Source: CAD feature listing. Evaluate the final solid. Frame: model axes, mm. A direction names the side the tool comes from. Round coordinates to 2 decimals unless told otherwise and drop trailing zeros. Write each loop counter-clockwise with the first axis right and the second up, starting at its lowest first coordinate (ties: lowest second). Pieces come first, ordered by that corner, then holes. Notation, with made-up numbers: (-11.5, -14) -> (5.5, -14) arc R28 ccw to (5.5, 12) -> close; hole circle Ø6 at (-15, 69). An arc over 180 degrees is marked (long way). Put each result on its own line as item: value.
```python
from build123d import *

# Parameters (mm, degrees)
SKETCH2_R          = 1.5875
CUT_EXTRUDE1_DEPTH = 13.7


with BuildPart() as part:
    # Sketch1 → Revolve1 (revolve)
    with BuildSketch(Plane.XY):
        with BuildLine():
            Line((12.7, 25.4), (17.4625, 25.4))
            ThreePointArc((17.4625, 25.4), (18.585032015, 24.935032015), (19.05, 23.8125))
            Line((19.05, 23.8125), (19.05, 14.2875))
            ThreePointArc((19.05, 14.2875), (19.514967985, 13.164967985), (20.6375, 12.7))
            Line((20.6375, 12.7), (33.3375, 12.7))
            ThreePointArc((33.3375, 12.7), (34.460032015, 12.235032015), (34.925, 11.1125))
            Line((34.925, 11.1125), (34.925, 0))
            Line((34.925, 0), (25.4, 0))
            Line((25.4, 0), (25.4, 3.175))
            ThreePointArc((25.4, 3.175), (24.47006403, 5.42006403), (22.225, 6.35))
            Line((22.225, 6.35), (12.7, 6.35))
            Line((12.7, 6.35), (12.7, 25.4))
        make_face()
    revolve(axis=Axis((0, 0, 0), (0, 1, 0)))

    # Sketch2 → Cut-Extrude1 (cut, through all)
    with BuildSketch(Plane(origin=(0, 12.7, 0), x_dir=(1, 0, 0), z_dir=(0, 1, 0))):
        with Locations((-21.328108288, 21.328108288)):
            Circle(SKETCH2_R)
        with Locations((21.328108288, 21.328108288)):
            Circle(SKETCH2_R)
        with Locations((21.328108288, -21.328108288)):
            Circle(SKETCH2_R)
        with Locations((-21.328108288, -21.328108288)):
            Circle(SKETCH2_R)
    extrude(amount=-CUT_EXTRUDE1_DEPTH, mode=Mode.SUBTRACT)


solid = part.part
```
Q1. Pin query (flat end, axial travel): pin 1 (1 mm diameter, centred on x = 4.5, z = -21, fed in from +Y); pin 2 (3 mm diameter, centred on x = -2.5, y = 8.5, fed in from -Z); pin 3 (3 mm diameter, centred on y = 11, z = 3.5, fed in from -X). Return the tip coordinate at first contact, or that it passes through.
Ans:
pin 1: stops at y = 12.7
pin 2: stops at z = -34.91
pin 3: stops at x = -34.87
Q2. Reachability of faces 4 (the flat face through (-1, 25.4, 13)), 5 (the flat face through (10, 6.35, 10)) from +Z, -Z, +X, -X, +Y, -Y: full face, straight path, thin tool, end or side. Return the list, or none.
Ans:
face 4: +Z, -Z, +X, -X, +Y
face 5: -Y
Q3. Cut plane C-C on y = 22.5. Output: boundary loops of the cut face in (x, z).
Ans:
outline: circle Ø38.1 at (0, 0); hole circle Ø25.4 at (0, 0)
Q4. Material intervals for line 1 (X direction, y = 16.25, z = -0.5); line 2 (Z direction, x = 0, y = 1.55) (3 decimals); line 3 (Y direction, x = -0.5, z = -31.5), sorted ascending. Write a range as [from, to].
Ans:
line 1: x = [-19.04, -12.69], [12.69, 19.04]
line 2: z = [-34.925, -25.4], [25.4, 34.925]
line 3: y = [0, 12.7]
Q5. Draft query along Z for faces 1 (the cylindrical face through (-22.5, 6.4, -22.4)), 2 (the flat face through (15.3, 12.7, 14.3)), 3 (the cylindrical face through (-15.12, 18.98, 11.59)). Return one class per face: +Z half, -Z half, draft (parallel to the pull), parting line (faces both ways), or undercut.
Ans:
face 1: undercut
face 2: draft
face 3: parting line
